Work out the finished part from the listing and answer in its coordinate system (mm). Give positions to 0.01 mm unless a question says otherwise; leave off trailing zeros. Loops run counter-clockwise (first coordinate to the right, second up) from the corner with the lowest first, then second, coordinate; pieces in that order, holes last. Notation, with made-up numbers: M 82.25,3.5 L 131.25,3.5 A28 ccw 131.25,22.5 Z; hole C -15,-13 d5. An arc over 180 degrees is marked long. Write item = value, one per line. Start each with the question number.
1. Consider L1, parallel to Z at x = 20, y = 89; L2, parallel to Y at x = 42.5, z = 20. Determine where each line is inside the solid, lowest interval first. Write a range as [from, to].
2. Section B-B on z = -34.5 is taken. Determine the outline of the cut face in (x, y).
3. Section A-A on y = 24 is taken. Determine the outline of the cut face in (x, z), plus the area to 3 significant figures.
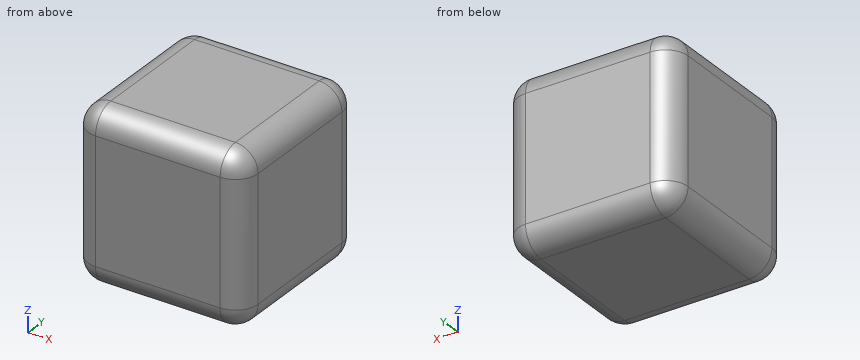
```python
from build123d import *

# Parameters (mm, degrees)
SKETCH1_W           = 150
SKETCH1_H           = 150
BOSS_EXTRUDE1_DEPTH = 150
FILLET1_R           = 20
SHELL1_T            = 1.5


with BuildPart() as part:
    # Sketch1 → Boss-Extrude1 (new body)
    with BuildSketch(Plane(origin=(0, 0, 0), x_dir=(1, 0, 0), z_dir=(0, 1, 0))):
        Rectangle(SKETCH1_W, SKETCH1_H)
    extrude(amount=BOSS_EXTRUDE1_DEPTH)

    # Fillet1
    fillet1_edges = [part.edges().sort_by_distance(p)[0] for p in [
        (75, 150, 0),
        (0, 150, -75),
        (-75, 150, 0),
        (0, 0, -75),
        (75, 0, 0),
        (0, 0, 75),
        (-75, 0, 0),
        (-75, 75, -75),
        (75, 75, -75),
        (75, 75, 75),
        (-75, 75, 75),
        (0, 150, 75),
    ]]
    fillet(fillet1_edges, radius=FILLET1_R)

    # Shell1 (no face opened: a closed hollow body)
    add(offset(amount=-SHELL1_T, mode=Mode.PRIVATE), mode=Mode.SUBTRACT)


solid = part.part
```
Verdict:
q1.L1 = [-75, -73.5], [73.5, 75]
q1.L2 = [0, 1.5], [148.5, 150]
q2.outline = M -75,20 A20 ccw -55,0 L 55,0 A20 ccw 75,20 L 75,130 A20 ccw 55,150 L -55,150 A20 ccw -75,130 Z; hole M -73.5,20 A18.5 ccw -55,1.5 L 55,1.5 A18.5 ccw 73.5,20 L 73.5,130 A18.5 ccw 55,148.5 L -55,148.5 A18.5 ccw -73.5,130 Z
q3.outline = M -75,-55 A20 ccw -55,-75 L 55,-75 A20 ccw 75,-55 L 75,55 A20 ccw 55,75 L -55,75 A20 ccw -75,55 Z; hole M -73.5,-55 A18.5 ccw -55,-73.5 L 55,-73.5 A18.5 ccw 73.5,-55 L 73.5,55 A18.5 ccw 55,73.5 L -55,73.5 A18.5 ccw -73.5,55 Z
q3.area = 841 mm2
